Input: part model. Units: mm. Frame: model coordinates. Round coordinates to 2 decimals unless told otherwise and drop trailing zeros. Loops run counter-clockwise (first coordinate to the right, second up) from the corner with the lowest first, then second, coordinate; pieces in that order, holes last. Notation, with made-up numbers: (9.5, -22) - (14.5, -22) arc R20 cw to (14.5, -4) - close; hole circle Ø7 at (-39, 35). An arc over 180 degrees is marked (long way). One line per question, with ' | ' between items. Start each with the question number.
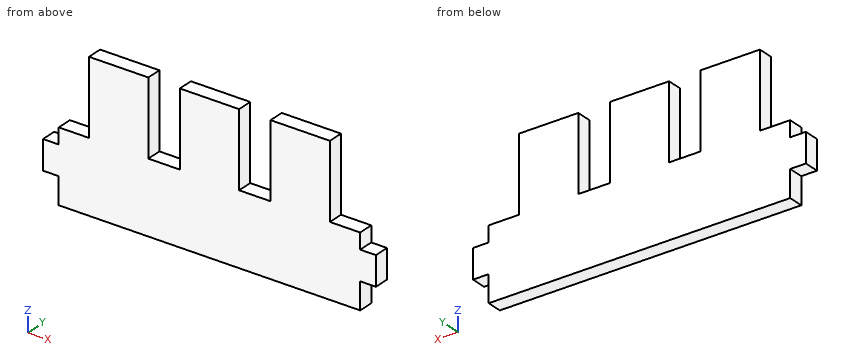
from build123d import *

# Parameters (mm, degrees)
SKETCH1_W           = 139.7
SKETCH1_H           = 57.15
BOSS_EXTRUDE1_DEPTH = 6.35
SKETCH3_W           = 24.892
SKETCH3_H           = 31.242
BOSS_EXTRUDE2_DEPTH = 6.35
SKETCH4_W           = 13.208
SKETCH4_H           = 13.208
CUT_EXTRUDE2_DEPTH  = 93.181443301
SKETCH5_W           = 295.464136086
SKETCH5_H           = 12.7
CUT_EXTRUDE3_DEPTH  = 93.181443301
SKETCH6_W           = 139.7
SKETCH6_H           = 12.446
BOSS_EXTRUDE3_DEPTH = 6.35
SKETCH7_W           = 139.7
SKETCH7_H           = 14.45
CUT_EXTRUDE4_DEPTH  = 93.181443301


with BuildPart() as part:
    # Sketch1 → Boss-Extrude1 (new body)
    with BuildSketch(Plane(origin=(0, 0, 0), x_dir=(1, 0, 0), z_dir=(0, 1, 0))):
        Rectangle(SKETCH1_W, SKETCH1_H)
    extrude(amount=BOSS_EXTRUDE1_DEPTH)

    # Sketch3 → Boss-Extrude2 (add)
    with BuildSketch(Plane(origin=(0, 0, 0), x_dir=(1, 0, 0), z_dir=(0, 1, 0))):
        with Locations((-38.1, -44.196)):
            Rectangle(SKETCH3_W, SKETCH3_H)
        with Locations((0, -44.196)):
            Rectangle(SKETCH3_W, SKETCH3_H)
        with Locations((38.1, -44.196)):
            Rectangle(SKETCH3_W, SKETCH3_H)
    extrude(amount=BOSS_EXTRUDE2_DEPTH)

    # Sketch4 → Cut-Extrude2 (cut, through all)
    with BuildSketch(Plane(origin=(0, 0, 0), x_dir=(1, 0, 0), z_dir=(0, 1, 0))):
        with Locations((69.85, 22.225)):
            Rectangle(SKETCH4_W, SKETCH4_H)
        with Locations((-69.85, -28.575)):
            Rectangle(SKETCH4_W, SKETCH4_H)
        with Locations((69.85, -3.175)):
            Rectangle(SKETCH4_W, SKETCH4_H)
        with Locations((69.85, -28.575)):
            Rectangle(SKETCH4_W, SKETCH4_H)
        with Locations((-69.85, -3.175)):
            Rectangle(SKETCH4_W, SKETCH4_H)
        with Locations((-69.85, 22.225)):
            Rectangle(SKETCH4_W, SKETCH4_H)
    extrude(amount=CUT_EXTRUDE2_DEPTH, mode=Mode.SUBTRACT)

    # Sketch5 → Cut-Extrude3 (cut, through all)
    with BuildSketch(Plane(origin=(0, 6.35, 0), x_dir=(1, 0, 0), z_dir=(0, 1, 0))):
        with Locations((7.963252738, 22.225)):
            Rectangle(SKETCH5_W, SKETCH5_H)
    extrude(amount=-CUT_EXTRUDE3_DEPTH, mode=Mode.SUBTRACT)

    # Sketch6 → Boss-Extrude3 (add)
    with BuildSketch(Plane(origin=(0, 6.35, 0), x_dir=(1, 0, 0), z_dir=(0, 1, 0))):
        with Locations((0, 9.652)):
            Rectangle(SKETCH6_W, SKETCH6_H)
    extrude(amount=-BOSS_EXTRUDE3_DEPTH)

    # Sketch7 → Cut-Extrude4 (cut, through all)
    with BuildSketch(Plane(origin=(0, 6.35, 0), x_dir=(1, 0, 0), z_dir=(0, 1, 0))):
        with Locations((0, 8.65)):
            Rectangle(SKETCH7_W, SKETCH7_H)
    extrude(amount=-CUT_EXTRUDE4_DEPTH, mode=Mode.SUBTRACT)


solid = part.part
(1) Section A-A, the plane z = 42.5. Output: boundary loops of the cut face in (x, y), plus the area to 3 significant figures.
(2) Pin query (flat end, axial travel): P1, Ø1.9, axis at y = 3, z = 44, coming from the +X side; P2, Ø1.9, axis at y = 4.5, z = 24, coming from the -X side; P3, Ø5, axis at x = -6.5, z = 13, coming from the -Y side; P4, Ø3, axis at y = 2.5, z = 41, coming from the -X side. Return the tip coordinate at first contact, or that it passes through.
(3) Line query: line 1 along X through (y, z) = (5, 56); line 2 along Z through (x, y) = (15, 3.25) (3 decimals); line 3 along X through (y, z) = (4.75, 8.5). Output: solid intervals per line, ascending. Write a range as from..to.
(4) Section B-B, the plane y = 5. Output: boundary loops of the cut face in (x, z) (3 decimals).
(5) Section C-C, the plane x = -52. Output: boundary loops of the cut face in (y, z) (3 decimals), plus the area to 4 significant figures.
(6) Section D-D, the plane z = 3. Output: boundary loops of the cut face in (x, y), plus the area to 3 significant figures.
Derived:
1) outline: (-50.55, 0) - (-25.65, 0) - (-25.65, 6.35) - (-50.55, 6.35) - close; (-12.45, 0) - (12.45, 0) - (12.45, 6.35) - (-12.45, 6.35) - close; (25.65, 0) - (50.55, 0) - (50.55, 6.35) - (25.65, 6.35) - close | area: 474 mm²
2) P1: stops at x = 50.55 | P2: stops at x = -63.25 | P3: stops at y = 0 | P4: stops at x = -50.55
3) line 1: x = -50.55..-25.65, -12.45..12.45, 25.65..50.55 | line 2: z = -1.425..28.575 | line 3: x = -63.25..63.25
4) outline: (-69.85, 9.779) - (-63.246, 9.779) - (-63.246, -1.425) - (63.246, -1.425) - (63.246, 9.779) - (69.85, 9.779) - (69.85, 21.971) - (63.246, 21.971) - (63.246, 28.575) - (50.546, 28.575) - (50.546, 59.817) - (25.654, 59.817) - (25.654, 28.575) - (12.446, 28.575) - (12.446, 59.817) - (-12.446, 59.817) - (-12.446, 28.575) - (-25.654, 28.575) - (-25.654, 59.817) - (-50.546, 59.817) - (-50.546, 28.575) - (-63.246, 28.575) - (-63.246, 21.971) - (-69.85, 21.971) - close
5) outline: (0, -1.425) - (6.35, -1.425) - (6.35, 28.575) - (0, 28.575) - close | area: 190.5 mm²
6) outline: (-63.25, 0) - (63.25, 0) - (63.25, 6.35) - (-63.25, 6.35) - close | area: 803 mm²
